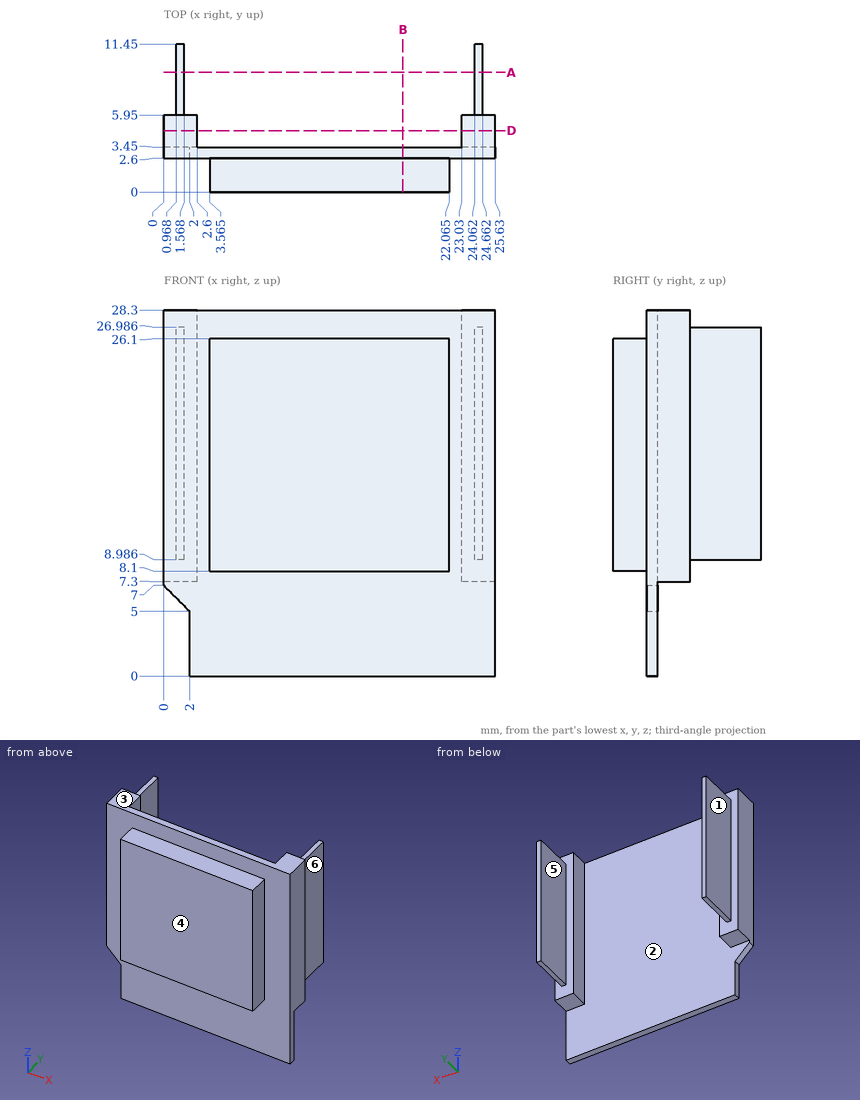
Can you work these out from the drawing? Everything is in mm from the part's minimum corner. A direction names the side the tool comes from. Round coordinates to 2 decimals unless told otherwise and drop trailing zeros. Order: outer loops, then holes, each group sorted by start corner. A loop starts at its lowest first (then second) coordinate and runs counter-clockwise, first axis right, second up. Notation, with made-up numbers: (37.5, -39.75) - (57.5, -39.75) arc R14 cw to (57.5, -27.75) - close; hole circle Ø10 at (-37.5, 68). An arc over 180 degrees is marked (long way). Answer in a Markdown table with one row per item.
(1) Please list where these lines run through material, in increasing order: L1, parallel to X at y = 10, z = 10; L2, parallel to X at y = 4.5, z = 24.25; L3, parallel to Y at x = 4, z = 23.25. Write a range as from..to.
From the geometry:
| item | result |
|---|---|
| L1 | x = 0.97..1.57, 24.06..24.66 |
| L2 | x = 0..2.6, 23.03..25.63 |
| L3 | y = 0..3.45 |
(2) Suppose I cut it at B-B, the plane x = 18.5. Please give me the cut outline in (y, z).
From the geometry:
| item | result |
|---|---|
| outline | (0, 8.1) - (2.6, 8.1) - (2.6, 0) - (3.45, 0) - (3.45, 28.3) - (2.6, 28.3) - (2.6, 26.1) - (0, 26.1) - close |
(3) If we mould it in two halves opening along X, with no side actions, what happens to the marked faces 1, 2 and 3? For each: released by +X, released by -X, zero draft, split by the parting line, or undercut.
From the geometry:
| item | result |
|---|---|
| face 1 | released by -X |
| face 2 | undercut |
| face 3 | zero draft |
(4) Suppose I cut it at D-D, the plane y = 4.75. Please give me the cut outline in (x, z), plus the area to 3 significant figures.
From the geometry:
| item | result |
|---|---|
| outline | (0, 7.3) - (2.6, 7.3) - (2.6, 28.3) - (0, 28.3) - close; (23.03, 7.3) - (25.63, 7.3) - (25.63, 28.3) - (23.03, 28.3) - close |
| area | 109 mm2 |
(5) Which directions (+Z, -Z, +X, -X, +Y, -Y) give clear straight access to the entire face, cutting with the end or side of a thin tool? Please do the marked faces 4, 5 and 6.
From the geometry:
| item | result |
|---|---|
| face 4 | +Z, -Z, +X, -X, -Y |
| face 5 | +Z, -Z, +Y |
| face 6 | +Z, -Z, +X, +Y |
(6) For P1, Ø6, axis at y = 9, z = 16.5, coming from the +X side; P2, Ø4.5, axis at y = 10, z = 15.5, coming from the -X side; P3, Ø1.3, axis at y = 1, z = 16.5, coming from the +X side (3 decimals); P4, Ø6, axis at y = 7.5, z = 22, coming from the -X side, each with a flat end and sliding along its axis, tell me the tip position at first contact or that it passes through.
From the geometry:
| item | result |
|---|---|
| P1 | stops at x = 24.66 |
| P2 | stops at x = 0.97 |
| P3 | stops at x = 22.065 |
| P4 | stops at x = 0 |
(7) Suppose I cut it at A-A, the plane y = 9.25. Please give me the cut outline in (x, z), plus the area to 3 significant figures.
From the geometry:
| item | result |
|---|---|
| outline | (0.97, 8.99) - (1.57, 8.99) - (1.57, 26.99) - (0.97, 26.99) - close; (24.06, 8.99) - (24.66, 8.99) - (24.66, 26.99) - (24.06, 26.99) - close |
| area | 21.6 mm2 |
